from build123d import *

# Parameters (mm, degrees)
ESQUISSE1_W             = 90
ESQUISSE1_H             = 19.7
BOSS_EXTRU_1_DEPTH      = 90
ENL_V_MAT_EXTRU_1_DEPTH = 30


with BuildPart() as part:
    # Esquisse1 → Boss.-Extru.1 (new body)
    with BuildSketch(Plane.XY):
        with Locations((-4.101935153, 9.85)):
            Rectangle(ESQUISSE1_W, ESQUISSE1_H)
    extrude(amount=BOSS_EXTRU_1_DEPTH)

    # Esquisse2 → Enlèv. mat.-Extru.1 (cut)
    with BuildSketch(Plane(origin=(0, 19.7, 0), x_dir=(1, 0, 0), z_dir=(0, 1, 0))):
        with BuildLine():
            Line((-34.101935153, -40), (-34.101935153, -90))
            Line((-34.101935153, -90), (25.898064847, -90))
            Line((25.898064847, -90), (25.898064847, -40))
            ThreePointArc((25.898064847, -40), (-4.101935153, -10), (-34.101935153, -40))
        make_face()
    extrude(amount=-ENL_V_MAT_EXTRU_1_DEPTH, mode=Mode.SUBTRACT)


solid = part.part
Part model, mm, in its own coordinate system. A direction names the side the tool comes from. Give positions to 0.01 mm unless a question says otherwise; leave off trailing zeros. Write each loop counter-clockwise with the first axis right and the second up, starting at its lowest first coordinate (ties: lowest second). Pieces come first, ordered by that corner, then holes.
1) Probe L1, parallel to X at y = 8.75, z = 59.5; L2, parallel to Z at x = -28.5, y = 16.5; L3, parallel to Z at x = -3, y = 19. List the from-to ranges inside material, lowest first.
Resolved:
L1: x = -49.1 to -34.1, 25.9 to 40.9
L2: z = 0 to 22.54
L3: z = 0 to 10.02
2) Two-plate mould, pull along X, no slides. Class faces 3 (the face through (25.898, 10, 65)), 4 (the face through (-35, 0, 34)), 5 (the face through (-49.102, 10, 44)): released by +X, released by -X, zero draft, split by the parting line, or undercut.
Resolved:
face 3: undercut
face 4: zero draft
face 5: released by -X
3) Cut at C-C on z = 17. Write the cut outline in (x, y).
Resolved:
outline: (-49.1, 0) - (-23.36, 0) - (-23.36, 19.7) - (-49.1, 19.7) - close; (15.16, 0) - (40.9, 0) - (40.9, 19.7) - (15.16, 19.7) - close
4) Cut at D-D on x = 18. Write the cut outline in (y, z), then the cut area to 3 significant figures.
Resolved:
outline: (0, 0) - (19.7, 0) - (19.7, 19.71) - (0, 19.71) - close
area: 388 mm2
5) Cut at B-B on y = 16.25. Write the cut outline in (x, z), then the cut area to 3 significant figures.
Resolved:
outline: (-49.1, 0) - (40.9, 0) - (40.9, 90) - (25.9, 90) - (25.9, 40) arc R30 cw to (-34.1, 40) - (-34.1, 90) - (-49.1, 90) - close
area: 3,690 mm2
6) Cut at A-A on z = 63. Write the cut outline in (x, y).
Resolved:
outline: (-49.1, 0) - (-34.1, 0) - (-34.1, 19.7) - (-49.1, 19.7) - close; (25.9, 0) - (40.9, 0) - (40.9, 19.7) - (25.9, 19.7) - close
7) Which spindle directions (+Z, -Z, +X, -X, +Y, -Y) get a long thin tool onto all of the face, cutting with end or side? Do faces 1 (the face through (40.898, 10, 44)), 2 (the face through (-34.102, 10, 65)). Say none if no direction does.
Resolved:
face 1: +Z, -Z, +X, +Y, -Y
face 2: +Z, +Y, -Y
8) Pin check, flat tip, straight feed: pin 1 (1 mm diameter, centred on x = 17, y = 8, fed in from +Z). Stop position of the tip, or through.
Resolved:
pin 1: stops at z = 19.18
